Geometry: see drawing. Coordinates: mm, zero at the bounding-box minimum. A direction names the side the tool comes from. Give positions to 0.01 mm unless a question says otherwise; leave off trailing zeros. Write each loop counter-clockwise with the first axis right and the second up, starting at its lowest first coordinate (ties: lowest second). Pieces come first, ordered by that corner, then holes. Notation, with made-up numbers: (83, -24) -> (116, -24) arc R8 ccw to (116, -19) -> close; hole circle Ø7 at (-16.5, -36.5). An arc over 180 degrees is marked (long way). Write item = value, one per line.
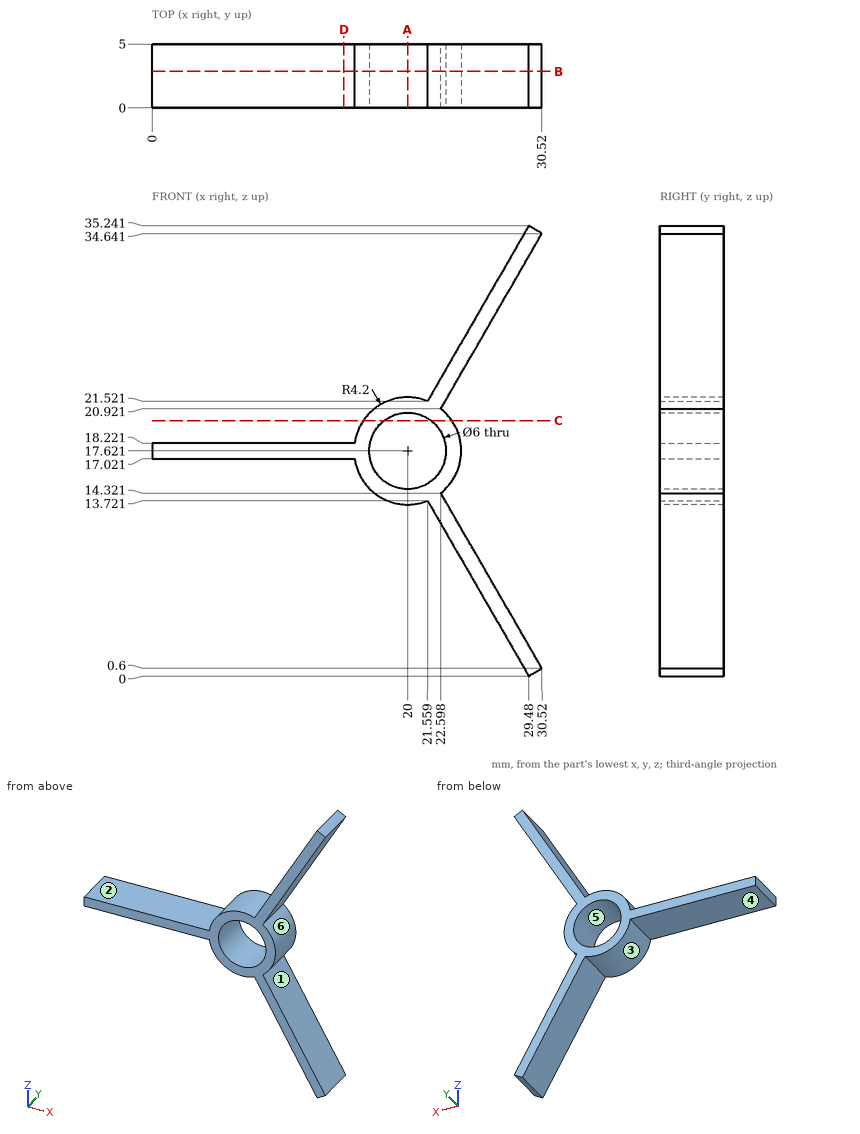
(1) First-contact query: pin 1 (3 mm diameter, centred on y = 2, z = 8, fed in from +X); pin 2 (1.5 mm diameter, centred on x = 9, y = 2, fed in from -Z); pin 3 (3 mm diameter, centred on y = 3.5, z = 29.5, fed in from +X). Flat tips, straight axial feed; report the tip coordinate or a pass-through.
Values follow:
pin_1 = 27.11
pin_2 = 17.02
pin_3 = 28.42
(2) Section query D-D (x = 15). Return loops of the section in (y, z).
Values follow:
outline = (0, 17.02) -> (5, 17.02) -> (5, 18.22) -> (0, 18.22) -> close
(3) Access query for the marked faces 1, 2 and 3. Directions: +Z, -Z, +X, -X, +Y, -Y. A direction counts if a zero-diameter tool reaches every point of the face in a straight line with its end or side. Return the directions, or none.
Values follow:
face_1 = +X, +Y, -Y
face_2 = +Z, -X, +Y, -Y
face_3 = -Z, +Y, -Y
(4) Material intervals for line 1 (Z direction, x = 10.5, y = 1.2); line 2 (Z direction, x = 18, y = 4.7) (1 decimal); line 3 (X direction, y = 3.3, z = 16.5), sorted ascending.
Values follow:
line_1 = 17.02 to 18.22
line_2 = 13.9 to 15.4, 19.9 to 21.3
line_3 = 15.95 to 17.22, 22.78 to 24.05
(5) Section query A-A (x = 20). Return loops of the section in (y, z).
Values follow:
outline = (0, 13.42) -> (5, 13.42) -> (5, 14.62) -> (0, 14.62) -> close; (0, 20.62) -> (5, 20.62) -> (5, 21.82) -> (0, 21.82) -> close
(6) Section query B-B (y = 2.85). Return loops of the section in (x, z).
Values follow:
outline = (0, 17.02) -> (15.84, 17.02) arc R4.2 ccw to (21.56, 13.72) -> (29.48, 0) -> (30.52, 0.6) -> (22.6, 14.32) arc R4.2 ccw to (22.6, 20.92) -> (30.52, 34.64) -> (29.48, 35.24) -> (21.56, 21.52) arc R4.2 ccw to (15.84, 18.22) -> (0, 18.22) -> close; hole circle Ø6 at (20, 17.62)
(7) Pull-direction query (X, two-part tool) for the marked faces 4, 5 and 6; classes: pulls with the +X half, pulls with the -X half, needs draft (parallel to the pull), parting line crosses it, or undercut.
Values follow:
face_4 = needs draft
face_5 = undercut
face_6 = pulls with the +X half
(8) Section query C-C (z = 20). Return loops of the section in (x, y).
Values follow:
outline = (16.54, 0) -> (18.17, 0) -> (18.17, 5) -> (16.54, 5) -> close; (21.83, 0) -> (23.46, 0) -> (23.46, 5) -> (21.83, 5) -> close
